Read the model definition and answer for the solid it produces. Units are mm, in the model's axes. A direction names the side the tool comes from. Give positions to 0.01 mm unless a question says otherwise; leave off trailing zeros. Order: outer loops, then holes, each group sorted by start corner. A loop starts at its lowest first (then second) coordinate and runs counter-clockwise, first axis right, second up. Notation, with made-up numbers: (-6, 21.5) - (32, 21.5) arc R26 cw to (32, 48.5) - close; hole circle Ø1 at (71, 2.5). An arc over 180 degrees is marked (long way). Return JSON: item names as keys, results as strings.
Autodesk Inventor part; units mm, degrees
ref_plane "YZ Plane" through (0, 0, 0) normal (1, 0, 0) x (0, 1, 0)
ref_plane "XZ Plane" through (0, 0, 0) normal (0, 1, 0) x (-1, 0, 0)
ref_plane "XY Plane" through (0, 0, 0) normal (0, 0, 1) x (1, 0, 0)
sketch "スケッチ1" plane through (0, 0, 0) normal (0, 0, 1) x (1, 0, 0)
  circle A0 centre (0, 0) radius 3
  circle A1 centre (0, 0) radius 1.5
  dimension "d0" = 6
  dimension "d1" = 3
extrude "押し出し1" add sketch "スケッチ1" along normal blind 35
fillet "フィレット1" radius 0.3 2 edges at (-3, 0, 35) (-3, 0, 0)
thread "ねじ1"
extrude "押し出し2" add sketch "スケッチ1" along normal blind 29 contours A1
extrude "押し出し3" cut sketch "スケッチ1" along normal blind 6 contours A1
thread "ねじ2"
properties part number "スペーサーM3L35アルミ" material "アルミニウム 2014-T4"
Q1. For faces 1 (the cylindrical face through (-1.5, -0.07, 2.96)), 2 (the cylindrical face through (-1.5, -0.07, 31.96)), 3 (the cylindrical face through (-3, 0, 17)), determine the directions among +Z, -Z, +X, -X, +Y, -Y from which every point of the face is accessible in a straight line to the end or side of a thin tool.
Values:
{"face 1": "-Z", "face 2": "+Z", "face 3": "+Z, -Z"}
Q2. Consider L1, parallel to Y at x = 0, z = 33.1; L2, parallel to Z at x = -1.25, y = 0; L3, parallel to Z at x = -2.25, y = -1.75. Determine where each line is inside the solid, lowest interval first.
Values:
{"L1": "y = -3 to -1.5, 1.5 to 3", "L2": "z = 6 to 29", "L3": "z = 0.04 to 34.96"}
Q3. A cutting plane is placed at C-C (z = 5). Write down the section's boundary in (x, y).
Values:
{"outline": "circle Ø6 at (0, 0); hole circle Ø3 at (0, 0)"}
Q4. Given pin 1 (2 mm diameter, centred on x = -1.5, y = -1, fed in from -Z); pin 2 (0.9 mm diameter, centred on x = 0.5, y = 0.5, fed in from -Z); pin 3 (2.5 mm diameter, centred on x = 0, y = 0, fed in from +Z), each flat-ended and moving along its own axis, determine where each tip first touches the part or whether it passes through.
Values:
{"pin 1": "stops at z = 0", "pin 2": "stops at z = 6", "pin 3": "stops at z = 29"}
Q5. A cutting plane is placed at A-A (y = 0). Write down the section's boundary in (x, z).
Values:
{"outline": "(-3, 0.3) arc R0.3 ccw to (-2.7, 0) - (-1.5, 0) - (-1.5, 6) - (1.5, 6) - (1.5, 0) - (2.7, 0) arc R0.3 ccw to (3, 0.3) - (3, 34.7) arc R0.3 ccw to (2.7, 35) - (1.5, 35) - (1.5, 29) - (-1.5, 29) - (-1.5, 35) - (-2.7, 35) arc R0.3 ccw to (-3, 34.7) - close"}
